from build123d import *

# Parameters (mm, degrees)
F1_DEPTH = 30
F3_DEPTH = 39.624


with BuildPart() as f1:
    # F0 (on Front) → F1 (new body)
    with BuildSketch(Plane.XZ):
        with BuildLine():
            ThreePointArc((68.123961, -37.994432), (79.922035, -27.327051), (89.973475, -15))
            Line((89.973475, -15), (3.805035, 25))
            Line((3.805035, 25), (-82.363405, -15))
            ThreePointArc((-82.363405, -15), (-72.311965, -27.327051), (-60.513891, -37.994432))
            Line((-60.513891, -37.994432), (-35.392356, -37.994432))
            Line((-35.392356, -37.994432), (3.805035, -15))
            Line((3.805035, -15), (43.002567, -37.994432))
            Line((43.002567, -37.994432), (68.123961, -37.994432))
        make_face()
    extrude(amount=F1_DEPTH)

    # F2 (on face) → F3 (cut)
    with BuildSketch(Plane(origin=(0, 0, -37.994432), x_dir=(1, 0, 0), z_dir=(0, 0, -1))):
        Polygon((0, 4), (26.541401, 4), (26.541401, 26), (-18.458599, 26), (-18.458599, 4), align=None)
    extrude(amount=-F3_DEPTH, mode=Mode.SUBTRACT)


solid = f1.part
Part model, mm, in its own coordinate system. A direction names the side the tool comes from. Coordinates: 2 decimals unless noted, no trailing zeros. Write each loop counter-clockwise with the first axis right and the second up, starting at its lowest first coordinate (ties: lowest second). Pieces come first, ordered by that corner, then holes. Notation, with made-up numbers: M 77,89 L 110,89 A24 cw 110,108 Z; hole C 65,82 d5. An arc over 180 degrees is marked long. Return JSON: item names as keys, results as strings.
1. Pull direction X, two halves, no side cores. Call faces 1 (the face through (-38.68, -14.79, 5.28)), 2 (the face through (-24.78, -14.79, -31.77)), 3 (the face through (3, 0, -13)): pulls with the +X half, pulls with the -X half, needs draft (parallel to the pull), parting line crosses it, or undercut.
Determined:
{"face 1": "pulls with the -X half", "face 2": "undercut", "face 3": "needs draft"}
2. Saw through at B-B, the plane z = -9. Write the cut outline in (x, y), then the cut area to 3 significant figures.
Determined:
{"outline": "M -69.44,-30 L 77.05,-30 L 77.05,0 L -69.44,0 Z; hole M -18.46,-26 L 26.54,-26 L 26.54,-4 L -18.46,-4 Z", "area": "3,400 mm²"}
3. 3-axis set-ups, long thin cutter, end or side, ignore diameter. For faces 4 (the face through (26.541, -15, -14)), 5 (the face through (31.84, -14.79, -31.446)), 6 (the face through (-48, -15, -37.994)): which of +Z, -Z, +X, -X, +Y, -Y reach the whole face in a straight line?
Determined:
{"face 4": "-Z", "face 5": "-Z, +Y, -Y", "face 6": "-Z, +X, -X, +Y, -Y"}
4. Saw through at A-A, the plane y = -19. Write the cut outline in (x, z), then the cut area to 3 significant figures.
Determined:
{"outline": "M -82.36,-15 A105 ccw -60.51,-37.99 L -35.39,-37.99 L -18.46,-28.06 L -18.46,1.63 L 26.54,1.63 L 26.54,-28.34 L 43,-37.99 L 68.12,-37.99 A105 ccw 89.97,-15 L 3.81,25 Z", "area": "5,010 mm²"}
5. Saw through at C-C, the plane x = -5. Write the cut outline in (y, z).
Determined:
{"outline": "M -30,-20.17 L -26,-20.17 L -26,1.63 L -4,1.63 L -4,-20.17 L 0,-20.17 L 0,20.91 L -30,20.91 Z"}
6. Flat gauge pins, fed straight in: pin 1 Ø1 at (y, z) = (-19.5, 18) entering from +X; pin 2 Ø6 at (x, y) = (6.5, -16) entering from -Z; pin 3 Ø12 at (x, y) = (-46.5, -18) entering from +Z. Where does each tip first touch, or does it go through?
Determined:
{"pin 1": "x = 19.96", "pin 2": "z = 1.63", "pin 3": "z = 4.43"}
7. Probe L1, parallel to Y at x = -2, z = 1.5; L2, parallel to X at y = -22.5, z = -7; L3, parallel to X at y = -25.75, z = -1.5. List the from-to ranges inside material, lowest first.
Determined:
{"L1": "-30 to -26, -4 to 0", "L2": "-65.13 to -18.46, 26.54 to 72.74", "L3": "-53.28 to -18.46, 26.54 to 60.89"}
8. Saw through at D-D, the plane z = -0.5. Write the cut outline in (x, y).
Determined:
{"outline": "M -51.13,-30 L 58.74,-30 L 58.74,0 L -51.13,0 Z; hole M -18.46,-26 L 26.54,-26 L 26.54,-4 L -18.46,-4 Z"}
